from build123d import *

# Parameters (mm, degrees)
BOSS_EXTRUDE1_DEPTH = 7
SKETCH2_R           = 2.75
CUT_EXTRUDE1_DEPTH  = 56.14752941
SKETCH3_R           = 7.1
CUT_EXTRUDE2_DEPTH  = 5
CUT_EXTRUDE3_REACH  = 57.148
SKETCH6_R           = 1.7
SKETCH9_W           = 30
SKETCH9_H           = 11
BOSS_EXTRUDE2_DEPTH = 18
SKETCH12_R          = 1.5
CUT_EXTRUDE5_DEPTH  = 61.143578211
CHAMFER2_SIZE       = 1
BOSS_EXTRUDE3_DEPTH = 5
CUT_EXTRUDE6_DEPTH  = 58.586890869
BOSS_EXTRUDE4_START = 3
BOSS_EXTRUDE4_DEPTH = 3


with BuildPart() as part:
    # Sketch1 → Boss-Extrude1 (new body)
    with BuildSketch(Plane.XY):
        with BuildLine():
            Line((-28.559544782, -15.511363636), (-19.332614929, -32.5))
            ThreePointArc((-19.332614929, -32.5), (0, -44), (19.332614929, -32.5))
            Line((19.332614929, -32.5), (28.559544782, -15.511363636))
            ThreePointArc((28.559544782, -15.511363636), (0, 32.5), (-28.559544782, -15.511363636))
        make_face()
    extrude(amount=BOSS_EXTRUDE1_DEPTH)

    # Sketch2 → Cut-Extrude1 (cut, through all)
    with BuildSketch(Plane.XY.offset(7)):
        with Locations((0, -22)):
            Circle(SKETCH2_R)
    extrude(amount=-CUT_EXTRUDE1_DEPTH, mode=Mode.SUBTRACT)

    # Sketch3 → Cut-Extrude2 (cut)
    with BuildSketch(Plane.XY.offset(7)):
        with Locations((0, -22)):
            Circle(SKETCH3_R)
    extrude(amount=-CUT_EXTRUDE2_DEPTH, mode=Mode.SUBTRACT)

    # Sketch6 → Cut-Extrude3 (cut, up to next)
    with BuildSketch(Plane.XY.offset(7), mode=Mode.PRIVATE) as cut_extrude3_sk1:
        with Locations((-12, 15.95)):
            Circle(SKETCH6_R)
    cut_extrude3_tool1 = extrude(cut_extrude3_sk1.sketch, amount=-CUT_EXTRUDE3_REACH, mode=Mode.PRIVATE) & part.part
    # Sketch6 → Cut-Extrude3 (cut, up to next)
    with BuildSketch(Plane.XY.offset(7), mode=Mode.PRIVATE) as cut_extrude3_sk2:
        with Locations((12, 15.95)):
            Circle(SKETCH6_R)
    cut_extrude3_tool2 = extrude(cut_extrude3_sk2.sketch, amount=-CUT_EXTRUDE3_REACH, mode=Mode.PRIVATE) & part.part
    # Sketch6 → Cut-Extrude3 (cut, up to next)
    with BuildSketch(Plane.XY.offset(7), mode=Mode.PRIVATE) as cut_extrude3_sk3:
        with Locations((-12, -1.05)):
            Circle(SKETCH6_R)
    cut_extrude3_tool3 = extrude(cut_extrude3_sk3.sketch, amount=-CUT_EXTRUDE3_REACH, mode=Mode.PRIVATE) & part.part
    # Sketch6 → Cut-Extrude3 (cut, up to next)
    with BuildSketch(Plane.XY.offset(7), mode=Mode.PRIVATE) as cut_extrude3_sk4:
        with Locations((12, -1.05)):
            Circle(SKETCH6_R)
    cut_extrude3_tool4 = extrude(cut_extrude3_sk4.sketch, amount=-CUT_EXTRUDE3_REACH, mode=Mode.PRIVATE) & part.part
    add(cut_extrude3_tool1.solids().sort_by_distance((-12, 15.95, 7))[0], mode=Mode.SUBTRACT)
    add(cut_extrude3_tool2.solids().sort_by_distance((12, 15.95, 7))[0], mode=Mode.SUBTRACT)
    add(cut_extrude3_tool3.solids().sort_by_distance((-12, -1.05, 7))[0], mode=Mode.SUBTRACT)
    add(cut_extrude3_tool4.solids().sort_by_distance((12, -1.05, 7))[0], mode=Mode.SUBTRACT)

    # Sketch9 → Boss-Extrude2 (add)
    with BuildSketch(Plane.XY.offset(7)):
        with Locations((0, 7.45)):
            Rectangle(SKETCH9_W, SKETCH9_H)
    extrude(amount=BOSS_EXTRUDE2_DEPTH)

    # Sketch10 → Cut-Revolve1 (revolve, cut)
    with BuildSketch(Plane.XY.offset(18.5), mode=Mode.PRIVATE) as cut_revolve1_sk:
        Polygon((-10.364859929, -0.79478264), (-6.482574253, 13.694104755), (-9.259611003, 14.438209509), (-11.071344319, 7.676728725), (-9.260233395, 7.191443016), (-11.330785756, -0.535963595), align=None)
    revolve(cut_revolve1_sk.sketch.rotate(Axis((-10.364859929, -0.79478264, 18.5), (0.25881904510252135, 0.9659258262890681, 0)), 180), axis=Axis((-10.364859929, -0.79478264, 18.5), (0.25881904510252135, 0.9659258262890681, 0)), mode=Mode.SUBTRACT)

    # Sketch11 → Cut-Revolve2 (revolve, cut)
    with BuildSketch(Plane.XY.offset(13.5), mode=Mode.PRIVATE) as cut_revolve2_sk:
        Polygon((10.364859929, -0.79478264), (6.482574253, 13.694104755), (3.705537502, 12.95), (5.517270818, 6.188519216), (7.328381742, 6.673804926), (9.398934103, -1.053601685), align=None)
    revolve(cut_revolve2_sk.sketch.rotate(Axis((10.364859929, -0.79478264, 13.5), (-0.258819045102522, 0.965925826289068, 0)), 180), axis=Axis((10.364859929, -0.79478264, 13.5), (-0.258819045102522, 0.965925826289068, 0)), mode=Mode.SUBTRACT)

    # Sketch12 → Cut-Extrude5 (cut, through all)
    with BuildSketch(Plane(origin=(0, 0, 0), x_dir=(-1, 0, 0), z_dir=(0, 0, -1))):
        with Locations((-5.3, -33.55)):
            Circle(SKETCH12_R)
        with Locations((4.2, -33.55)):
            Circle(SKETCH12_R)
    extrude(amount=-CUT_EXTRUDE5_DEPTH, mode=Mode.SUBTRACT)

    # Chamfer2
    chamfer2_edges = [part.edges().sort_by_distance(p)[0] for p in [
        (6.8, -33.55, 0),
        (-2.7, -33.55, 0),
    ]]
    chamfer(chamfer2_edges, length=CHAMFER2_SIZE)

    # Sketch13 → Boss-Extrude3 (add, symmetric)
    with BuildSketch(Plane(origin=(0, 0, 0), x_dir=(0, 0, -1), z_dir=(1, 0, 0))):
        Polygon((-25, 1.95), (-7, -6), (-7, 1.95), align=None)
    extrude(amount=BOSS_EXTRUDE3_DEPTH, both=True)

    # Sketch14 → Cut-Extrude6 (cut, through all)
    with BuildSketch(Plane.XY.offset(7)):
        with BuildLine():
            Line((-22, 7.45), (-22, -22))
            ThreePointArc((-22, -22), (-21.322728817, -27.416755097), (-19.332614929, -32.5))
            Line((-19.332614929, -32.5), (-28.559544782, -15.511363636))
            ThreePointArc((-28.559544782, -15.511363636), (0, 32.5), (28.559544782, -15.511363636))
            Line((28.559544782, -15.511363636), (19.332614929, -32.5))
            ThreePointArc((19.332614929, -32.5), (21.322728817, -27.416755097), (22, -22))
            Line((22, -22), (22, 7.45))
            ThreePointArc((22, 7.45), (0, 29.45), (-22, 7.45))
        make_face()
    extrude(amount=-CUT_EXTRUDE6_DEPTH, mode=Mode.SUBTRACT)

    # Sketch15 → Boss-Extrude4 (add)
    with BuildSketch(Plane.XY.offset(7).offset(BOSS_EXTRUDE4_START)):
        with BuildLine():
            Line((-22, 7.45), (-22, -22))
            ThreePointArc((-22, -22), (0, -44), (22, -22))
            Line((22, -22), (22, 7.45))
            ThreePointArc((22, 7.45), (0, 29.45), (-22, 7.45))
        make_face()
        with BuildLine():
            Line((-18, 7.45), (-18, -22))
            ThreePointArc((-18, -22), (0, -40), (18, -22))
            Line((18, -22), (18, 7.45))
            ThreePointArc((18, 7.45), (0, 25.45), (-18, 7.45))
        make_face(mode=Mode.SUBTRACT)
    extrude(amount=-BOSS_EXTRUDE4_DEPTH)


solid = part.part
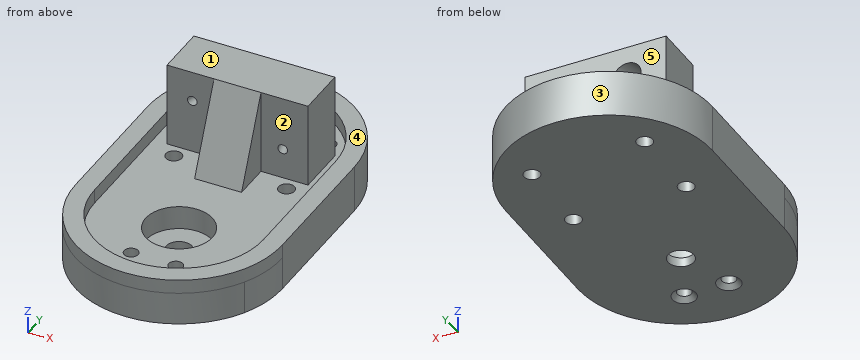
Source: CAD feature listing. Evaluate the final solid. Frame: model axes, mm. Face numbers are marked on the shaded views. A direction names the side the tool comes from. Give positions to 0.01 mm unless a question says otherwise; leave off trailing zeros. Order: outer loops, then holes, each group sorted by start corner. A loop starts at its lowest first (then second) coordinate and runs counter-clockwise, first axis right, second up. Notation, with made-up numbers: (-21.75, 71) -> (37.25, 71) arc R22 cw to (37.25, 105) -> close; hole circle Ø6 at (2.5, 14). An arc over 180 degrees is marked (long way). Write item = value, one per line.
Q1. Cut plane A-A, the plane z = 8.5. Output: boundary loops of the cut face in (x, y).
Data:
outline = (-22, -22) arc R22 ccw to (22, -22) -> (22, 7.45) arc R22 ccw to (-22, 7.45) -> close; (-15, 1.95) -> (-5, 1.95) -> (-5, -5.34) -> (5, -5.34) -> (5, 1.95) -> (15, 1.95) -> (15, 12.95) -> (-15, 12.95) -> close; hole (-18, -22) arc R18 ccw to (18, -22) -> (18, 7.45) arc R18 ccw to (-18, 7.45) -> close
Q2. Cut plane D-D, the plane y = -10.5. Output: boundary loops of the cut face in (x, z).
Data:
outline = (-22, 0) -> (22, 0) -> (22, 10) -> (18, 10) -> (18, 7) -> (-18, 7) -> (-18, 10) -> (-22, 10) -> close
Q3. Pull-direction query (Y, two-part tool) for the marked faces 3, 4 and 5; classes: released by +Y, released by -Y, zero draft, split by the parting line, or undercut.
Data:
face_3 = released by +Y
face_4 = zero draft
face_5 = undercut
Q4. Cut plane B-B, the plane x = 0. Output: boundary loops of the cut face in (y, z), and give its area (3 significant figures).
Data:
outline = (-44, 0) -> (-24.75, 0) -> (-24.75, 2) -> (-29.1, 2) -> (-29.1, 7) -> (-40, 7) -> (-40, 10) -> (-44, 10) -> close; (-19.25, 0) -> (29.45, 0) -> (29.45, 10) -> (25.45, 10) -> (25.45, 7) -> (12.95, 7) -> (12.95, 25) -> (1.95, 25) -> (-6, 7) -> (-14.9, 7) -> (-14.9, 2) -> (-19.25, 2) -> close
area = 726 mm^2
Q5. Cut plane C-C, the plane z = 5.25. Output: boundary loops of the cut face in (x, y).
Data:
outline = (-22, -22) arc R22 ccw to (22, -22) -> (22, 7.45) arc R22 ccw to (-22, 7.45) -> close; hole circle Ø3.4 at (-12, -1.05); hole circle Ø3.4 at (-12, 15.95); hole circle Ø14.2 at (0, -22); hole circle Ø3 at (-4.2, -33.55); hole circle Ø3 at (5.3, -33.55); hole circle Ø3.4 at (12, -1.05); hole circle Ø3.4 at (12, 15.95)
Q6. Set-up query: the marked faces 1 and 2. Return all of +Z, -Z, +X, -X, +Y, -Y with unobstructed straight access to the full face (end or side cutting, diameter ignored); none if empty.
Data:
face_1 = +Z, +X, -X, +Y, -Y
face_2 = +Z
Q7. Material intervals for line 1 (Y direction, x = 0, z = 5); line 2 (Y direction, x = -12, z = 2.5); line 3 (Z direction, x = 8.5, y = 6.5), sorted ascending. Write a range as from..to.
Data:
line_1 = -44..-29.1, -14.9..29.45
line_2 = -40.44..-2.75, 0.65..14.25, 17.65..25.89
line_3 = 0..12.5, 14.5..25
Q8. Pin query (flat end, axial travel): pin 1 (9 mm diameter, centred on x = 2, z = 16, fed in from +Y); pin 2 (4 mm diameter, centred on y = -1.5, z = 20, fed in from +X); pin 3 (3 mm diameter, centred on x = -12, z = 12.5, fed in from -Y); pin 4 (3 mm diameter, centred on x = -12, y = -1.05, fed in from -Z). Return the tip coordinate at first contact, or that it passes through.
Data:
pin_1 = 12.95
pin_2 = 5
pin_3 = 1.95
pin_4 = through
